Geometry check sheet. Reference: the model listing, model coordinates, mm. A direction names the side the tool comes from. Round coordinates to 2 decimals unless told otherwise and drop trailing zeros. Write each loop counter-clockwise with the first axis right and the second up, starting at its lowest first coordinate (ties: lowest second). Pieces come first, ordered by that corner, then holes. Notation, with made-up numbers: M 2.5,-17.75 L 53.5,-17.75 A25 ccw 53.5,10.25 Z; hole C -39,29.5 d8. An arc over 180 degrees is marked long. Use a Markdown table: item, result.
Autodesk Inventor part; units mm, degrees
ref_plane "YZ Plane" through (0, 0, 0) normal (1, 0, 0) x (0, 1, 0)
ref_plane "XZ Plane" through (0, 0, 0) normal (0, 1, 0) x (-1, 0, 0)
ref_plane "XY Plane" through (0, 0, 0) normal (0, 0, 1) x (1, 0, 0)
sketch "Sketch1" plane through (0, 0, 0) normal (0, 0, 1) x (1, 0, 0)
  line L0 (0, 50.8) -> (0, 0)
  line L1 (152.4, 0) -> (152.4, 0)
  line L2 (19.05, 0) -> (133.35, 0)
  line L3 (152.4, 0) -> (152.4, 50.8)
  line L4 (19.05, 50.8) -> (133.35, 50.8)
  line L5 (0, 50.8) -> (0, 69.85)
  line L6 (0, 69.85) -> (19.05, 69.85)
  line L7 (19.05, 69.85) -> (19.05, 50.8)
  line L8 (0, 0) -> (0, -19.05)
  line L9 (0, -19.05) -> (19.05, -19.05)
  line L10 (19.05, -19.05) -> (19.05, 0)
  line L11 (133.35, 50.8) -> (133.35, 69.85)
  line L12 (133.35, 69.85) -> (152.4, 69.85)
  line L13 (152.4, 69.85) -> (152.4, 50.8)
  line L14 (152.4, 0) -> (152.4, -19.05)
  line L15 (152.4, -19.05) -> (133.35, -19.05)
  line L16 (133.35, -19.05) -> (133.35, 0)
  dimension "d23" = 50.8
  dimension "d26" = 152.4
  dimension "d77" = 19.05
  dimension "d78" = 19.05
  dimension "d79" = 19.05
  dimension "d81" = 19.05
  dimension "d82" = 19.05
  dimension "d83" = 19.05
  dimension "d84" = 19.05
extrude "Plate2" add sketch "Sketch1" along normal blind 3.048
sketch "Sketch8" plane through (0, 0, 3.048) normal (0, 0, 1) x (1, 0, 0)
  line L0 (133.35, 0) -> (19.05, 0)
  line L1 (19.05, 50.8) -> (19.05, 0)
  line L2 (19.05, 25.4) -> (19.05, 44.45)
  line L3 (19.05, 25.4) -> (19.05, 6.35)
  circle A0 centre (19.05, 44.45) radius 1.9844
  circle A1 centre (19.05, 6.35) radius 1.9844
  line L4 (152.4, 69.85) -> (152.4, -19.05)
  circle A2 centre (133.35, 44.45) radius 1.9812
  circle A3 centre (133.35, 6.35) radius 1.9812
  line L5 (19.05, -19.05) -> (0, -19.05)
  line L6 (19.05, 0) -> (19.05, -19.05)
  line L7 (133.35, -19.05) -> (133.35, 0)
  line L8 (152.4, -19.05) -> (133.35, -19.05)
  line L9 (133.35, 69.85) -> (152.4, 69.85)
  line L10 (19.05, 69.85) -> (19.05, 50.8)
  line L11 (0, 69.85) -> (19.05, 69.85)
  circle A4 centre (9.525, 60.325) radius 3.3782
  circle A5 centre (9.525, -9.525) radius 3.3782
  circle A6 centre (142.875, 60.325) radius 3.3782
  circle A7 centre (142.875, -9.525) radius 3.3782
  point P0 (0, 0)
  point P1 (152.4, 0)
  point P2 (152.4, 50.8)
  dimension "d63" = 19.05
  dimension "d64" = 19.05
  dimension "d65" = 3.9688
  dimension "d66" = 3.9688
  dimension "d69" = 3.9624
  dimension "d70" = 3.9624
  dimension "d71" = 19.05
  dimension "d72" = 38.1
  dimension "d73" = 19.05
  dimension "d74" = 6.35
  dimension "d85" = 6.7564
  dimension "d86" = 6.7564
  dimension "d87" = 9.525
  dimension "d88" = 9.525
  dimension "d89" = 9.525
  dimension "d90" = 9.525
  dimension "d92" = 6.7564
  dimension "d93" = 6.7564
  dimension "d94" = 9.525
  dimension "d95" = 9.525
  dimension "d96" = 9.525
  dimension "d97" = 9.525
  dimension "d98" = 6.35
extrude "Cut9" cut sketch "Sketch8" against normal blind 3.048
equation "\"d105\" = Thickness"
equation "\"BendRadius\" = Thickness"
equation "\"BendReliefWidth\" = Thickness"
equation "\"BendReliefDepth\" = 0.5 * Thickness"
equation "\"CornerReliefSize\" = 4 * Thickness"
equation "\"MinimumRemnant\" = 2 * Thickness"
equation "\"TransitionRadius\" = BendRadius"
equation "\"JacobiRadiusSize\" = BendRadius"
equation "\"GapSize\" = Thickness"
equation "\"d10\" = BendRadius"
equation "\"d11\" = BendRadius"
properties part number "Pneumatic Piston Bracket_v1"
Item 1: Cross-section at A-A, the plane y = 6.35. Record the cut outline in (x, z).
Outcome:
| item | result |
|---|---|
| outline | M 0,0 L 17.07,0 L 17.07,3.05 L 0,3.05 Z; M 21.03,0 L 131.37,0 L 131.37,3.05 L 21.03,3.05 Z; M 135.33,0 L 152.4,0 L 152.4,3.05 L 135.33,3.05 Z |
Item 2: Go/stop test with flat-tipped pins: pin 1 (6 mm diameter, centred on x = 9.525, y = -9.525, fed in from -Z); pin 2 (0.9 mm diameter, centred on x = 62.5, z = 1.5, fed in from -Y); pin 3 (1 mm diameter, centred on x = 77.5, z = 2.5, fed in from +Y). Record where each tip stops, or that it passes through.
Outcome:
| item | result |
|---|---|
| pin 1 | passes through |
| pin 2 | stops at y = 0 |
| pin 3 | stops at y = 50.8 |
Item 3: Cross-section at B-B, the plane z = 1.95. Count the separate pieces of the cut face and the enclosed holes in it, and give its area (3 significant figures).
Outcome:
| item | result |
|---|---|
| separate pieces | 1 |
| enclosed holes | 8 |
| area | 9,000 mm2 |
Item 4: Material ranges on line 1 along X through (y, z) = (-10, 1.7); line 2 along X through (y, z) = (64, 0.65); line 3 along Y through (x, z) = (142.5, 2.6), recorded low to high. Write a range as from..to.
Outcome:
| item | result |
|---|---|
| line 1 | x = 0..6.18, 12.87..19.05, 133.35..139.53, 146.22..152.4 |
| line 2 | x = 0..19.05, 133.35..152.4 |
| line 3 | y = -19.05..-12.88, -6.17..56.97, 63.68..69.85 |
Item 5: Cross-section at C-C, the plane y = 62. Record the cut outline in (x, z), and give its area (3 significant figures).
Outcome:
| item | result |
|---|---|
| outline | M 0,0 L 6.59,0 L 6.59,3.05 L 0,3.05 Z; M 12.46,0 L 19.05,0 L 19.05,3.05 L 12.46,3.05 Z; M 133.35,0 L 139.94,0 L 139.94,3.05 L 133.35,3.05 Z; M 145.81,0 L 152.4,0 L 152.4,3.05 L 145.81,3.05 Z |
| area | 80.4 mm2 |
Item 6: Access from +Z, -Z, +X, -X, +Y, -Y to the whole of each face (thin tool, end or side, straight path). Record for faces 4 (the face through (19.05, -10, 2)), 5 (the face through (133.35, 60, 2)), 6 (the face through (135.24, 6.95, 1.55)).
Outcome:
| item | result |
|---|---|
| face 4 | +Z, -Z, -Y |
| face 5 | +Z, -Z, +Y |
| face 6 | +Z, -Z |
Item 7: Cross-section at D-D, the plane x = 34.5. Record the cut outline in (y, z), and give its area (3 significant figures).
Outcome:
| item | result |
|---|---|
| outline | M 0,0 L 50.8,0 L 50.8,3.05 L 0,3.05 Z |
| area | 155 mm2 |
Item 8: Mould release check, pull along Y, two halves, no side actions. Record for faces 1 (the face through (133.35, -10, 2)), 2 (the face through (143, 69.85, 2)), 3 (the face through (144.434, 57.328, 1.545)): +Y half, -Y half, draft (parallel to the pull), parting line (faces both ways), or undercut.
Outcome:
| item | result |
|---|---|
| face 1 | draft |
| face 2 | +Y half |
| face 3 | undercut |
